For this review, take the finished solid that the model builds, in its own axes (mm). Face numbers are marked on the shaded views. A direction names the side the tool comes from. Coordinates: 2 decimals unless noted, no trailing zeros. Order: outer loops, then holes, each group sorted by start corner. A loop starts at its lowest first (then second) coordinate and runs counter-clockwise, first axis right, second up. Notation, with made-up numbers: (32.5, 30.5) -> (45.5, 30.5) arc R24 cw to (45.5, 43.5) -> close; hole circle Ø6 at (-10, 14). An arc over 180 degrees is marked (long way). Return JSON: item names as keys, results as strings. Group by question number.
Item 1: Take a section at A-A (z = -109). Write out the cut boundary in (x, y).
Item 2: Insertion check: pin 1 (6 mm diameter, centred on x = -16, y = 5.5, fed in from +Z); pin 2 (4 mm diameter, centred on y = 4.5, z = -83.5, fed in from -X); pin 3 (8.5 mm diameter, centred on y = 8.47, z = -154, fed in from +X); pin 4 (8 mm diameter, centred on x = -7.5, y = 2, fed in from +Z). Each pin has a flat end and moves straight along its axis. Give the tip position at first contact, or say it passes through.
Item 3: Draft analysis for pull direction X (two halves, no side actions). For the marked faces 1, 2, 3 and 4, state which applies: +X half, -X half, draft (parallel to the pull), parting line (faces both ways), or undercut.
Item 4: For line 1 along X through (y, z) = (4.25, -148.5); line 2 along Y through (x, z) = (0, -137); line 3 along Z through (x, y) = (16, 5.5), list the stretches that pass through material, from the lowest coordinate up.
Item 5: Machinability: for the marked faces 5, 6, 7, 8 and 9, which of the approach directions +Z, -Z, +X, -X, +Y, -Y give a long, thin tool a straight path to every point of the face, cutting with its end or side? Answer none if there is none.
Item 6: Take a section at D-D (x = -11). Write out the cut boundary in (y, z), then the cut area to 3 significant figures.
Item 7: Take a section at B-B (z = -84). Count the separate pieces of the cut face and the enclosed holes in it, then the cut area to 3 significant figures.
Item 8: Take a section at C-C (z = -142). Write out the cut boundary in (x, y).
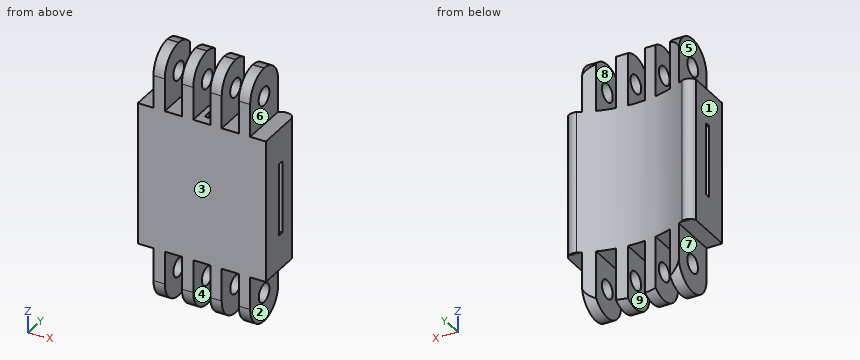
```python
from build123d import *

# Parameters (mm, degrees)
BOSS_EXTRUDE1_DEPTH = 20
CUT_EXTRUDE21_START = -45
CUT_EXTRUDE21_DEPTH = 45
CUT_EXTRUDE23_DEPTH = 444
SKETCH9_R           = 3.25
SKETCH9_R_2         = 3.15
CUT_EXTRUDE24_DEPTH = 45
CUT_EXTRUDE26_DEPTH = 444
CUT_EXTRUDE27_DEPTH = 45


# Read off the part's stored shape, not the designer's step: Cut-Extrude21
with BuildPart() as part:
    # Sketch1 → Boss-Extrude1 (new body)
    with BuildSketch(Plane(origin=(0, 0, 0), x_dir=(1, 0, 0), z_dir=(0, 1, 0))):
        Polygon((-17, 94), (-17, 74), (-15, 74), (-13, 74), (-13, 94), (-12.5, 94), (-7.5, 94), (-7, 94), (-7, 74), (-5, 74), (-3, 74), (-3, 94), (-2.5, 94), (2.5, 94), (3, 94), (3, 74), (5, 74), (7, 74), (7, 94), (7.5, 94), (12.5, 94), (13, 94), (13, 74), (17, 74), (17, 94), (17.5, 94), (22.5, 94), (22.5, 144), (17.5, 144), (17, 144), (17, 164), (15, 164), (13, 164), (13, 144), (12.5, 144), (7.5, 144), (7, 144), (7, 164), (5, 164), (3, 164), (3, 144), (2.5, 144), (-2.5, 144), (-3, 144), (-3, 164), (-5, 164), (-7, 164), (-7, 144), (-7.5, 144), (-12.5, 144), (-13, 144), (-13, 164), (-15, 164), (-17, 164), (-17, 144), (-17.5, 144), (-22.5, 144), (-22.5, 94), (-17.5, 94), align=None)
    extrude(amount=BOSS_EXTRUDE1_DEPTH)

    # Cut-Extrude21 outline → Cut-Extrude21 (cut)
    with BuildSketch(Plane(origin=(22.5, 0, 0), x_dir=(0, 0, -1), z_dir=(1, 0, 0)).offset(CUT_EXTRUDE21_START)):
        with BuildLine():
            Line((82.499126156, 17), (93.999126156, 17))
            Line((93.999126156, 17), (93.999126156, 20))
            Line((93.999126156, 20), (74, 20))
            Line((74, 20), (74, 8.62187939))
            ThreePointArc((74, 8.62187939), (76.531964972, 14.553345142), (82.499126156, 17))
        make_face()
        with BuildLine():
            Line((143.999126156, 20), (143.999126156, 17))
            Line((143.999126156, 17), (155.499126156, 17))
            ThreePointArc((155.499126156, 17), (163.999126156, 8.5), (155.499126156, 0))
            Line((155.499126156, 0), (164, 0))
            Line((164, 0), (164, 20))
            Line((164, 20), (143.999126156, 20))
        make_face()
        with BuildLine():
            ThreePointArc((82.499126156, 0), (76.531964972, 2.446654858), (74, 8.37812061))
            Line((74, 8.37812061), (74, 0))
            Line((74, 0), (82.499126156, 0))
        make_face()
    extrude(amount=CUT_EXTRUDE21_DEPTH, mode=Mode.SUBTRACT)

    # Sketch2 → Cut-Extrude23 (cut)
    with BuildSketch(Plane.XY.offset(50)):
        with BuildLine():
            Line((-22.5, 20), (22.5, 20))
            Line((22.5, 20), (22.5, 16))
            ThreePointArc((22.5, 16), (20.832845478, 17.631987193), (18.5, 17.607120136))
            ThreePointArc((18.5, 17.607120136), (0, 13.071891388), (-18.5, 17.607120136))
            ThreePointArc((-18.5, 17.607120136), (-20.832845478, 17.631987193), (-22.5, 16))
            Line((-22.5, 16), (-22.5, 20))
        make_face()
    extrude(amount=-CUT_EXTRUDE23_DEPTH, mode=Mode.SUBTRACT)

    # Sketch9 → Cut-Extrude24 (cut)
    with BuildSketch(Plane(origin=(22.5, 0, 0), x_dir=(0, 0, -1), z_dir=(1, 0, 0))):
        with Locations((153.999563078, 8.466039352)):
            Circle(SKETCH9_R)
        with Locations((84, 8.405099657)):
            Circle(SKETCH9_R)
        with Locations((178, 8.5)):
            Circle(SKETCH9_R_2)
        with Locations((60, 8.5)):
            Circle(SKETCH9_R_2)
    extrude(amount=-CUT_EXTRUDE24_DEPTH, mode=Mode.SUBTRACT)

    # Sketch12 → Cut-Extrude26 (cut)
    with BuildSketch(Plane.XY.offset(50)):
        Polygon((-1, 3.35), (-1, 6.55), (0, 6.55), (1, 6.55), (1, 3.35), align=None)
    extrude(amount=-CUT_EXTRUDE26_DEPTH, mode=Mode.SUBTRACT)

    # Sketch13 → Cut-Extrude27 (cut)
    with BuildSketch(Plane(origin=(22.5, 0, 0), x_dir=(0, 0, -1), z_dir=(1, 0, 0))):
        Polygon((119, 8), (131.7, 8), (131.7, 10), (106.3, 10), (106.3, 8), align=None)
    extrude(amount=-CUT_EXTRUDE27_DEPTH, mode=Mode.SUBTRACT)


solid = part.part
```
Findings below:
{
 "1": {"outline": "(-22.5, 0) -> (22.5, 0) -> (22.5, 8) -> (-22.5, 8) -> close; (-22.5, 10) -> (22.5, 10) -> (22.5, 16) arc R3.05 ccw to (18.5, 17.61) arc R40 cw to (-18.5, 17.61) arc R3.05 ccw to (-22.5, 16) -> close; hole (-1, 3.35) -> (1, 3.35) -> (1, 6.55) -> (-1, 6.55) -> close"},
 "2": {"pin 1": "stops at z = -74", "pin 2": "stops at x = -17", "pin 3": "stops at x = 17", "pin 4": "stops at z = -74.38"},
 "3": {"face 1": "-X half", "face 2": "+X half", "face 3": "draft", "face 4": "undercut"},
 "4": {"line 1": "x = -17 to -13, -7 to -3, 3 to 7, 13 to 17", "line 2": "y = 0 to 3.35, 6.55 to 13.07", "line 3": "z = -163.45 to -155.33, -152.67 to -85.46, -82.54 to -74.55"},
 "5": {"face 5": "+Z, -X, +Y, -Y", "face 6": "+Z, +X, +Y, -Y", "face 7": "-Z, -X, +Y, -Y", "face 8": "+Z, +Y, -Y", "face 9": "-Z, +Y, -Y"},
 "6": {"outline": "(0, -144) -> (14.61, -144) -> (14.61, -94) -> (0, -94) -> close; hole (8, -131.7) -> (10, -131.7) -> (10, -106.3) -> (8, -106.3) -> close", "area": "680 mm2"},
 "7": {"separate pieces": "8", "enclosed holes": "0", "area": "131 mm2"},
 "8": {"outline": "(-22.5, 0) -> (22.5, 0) -> (22.5, 16) arc R3.05 ccw to (18.5, 17.61) arc R40 cw to (-18.5, 17.61) arc R3.05 ccw to (-22.5, 16) -> close; hole (-1, 3.35) -> (1, 3.35) -> (1, 6.55) -> (-1, 6.55) -> close"}
}
